Autodesk Inventor part; units mm, degrees
ref_plane "YZ Plane" through (0, 0, 0) normal (1, 0, 0) x (0, 1, 0)
ref_plane "XZ Plane" through (0, 0, 0) normal (0, 1, 0) x (-1, 0, 0)
ref_plane "XY Plane" through (0, 0, 0) normal (0, 0, 1) x (1, 0, 0)
sketch "Sketch1" plane through (0, 0, 0) normal (0, 0, 1) x (1, 0, 0)
  circle A0 centre (0, 0) radius 22
  dimension "d0" = 44
extrude "Extrusion1" add sketch "Sketch1" along normal blind 2
sketch "Sketch2" plane through (0, 0, 2) normal (0, 0, 1) x (1, 0, 0)
  line L0 (-15, 0) -> (15, 0) construction
  point P0 (0, 0)
  point P1 (0, 0)
  dimension "d3" = 30
hole "Hole1" at (-15, 0, 2) at (15, 0, 2) direction (0, 0, -1) diameter 3.4 end through all
sketch "Sketch3" plane through (0, 0, 2) normal (0, 0, 1) x (1, 0, 0)
  line L0 (-9, 15) -> (9, 15)
  line L1 (9, 15) -> (9, -15)
  line L2 (9, -15) -> (-9, -15)
  line L3 (-9, -15) -> (-9, 15)
  line L4 (7.2, 13.2) -> (-7.2, 13.2)
  line L5 (-7.2, 13.2) -> (-7.2, -13.2)
  line L6 (-7.2, -13.2) -> (7.2, -13.2)
  line L7 (7.2, -13.2) -> (7.2, 13.2)
  point P0 (0, 0)
  point P1 (9, 0)
  point P2 (0, 15)
  dimension "d11" = 30
  dimension "d12" = 18
  dimension "d13" = 1.8
extrude "Extrusion2" cut sketch "Sketch3" against normal blind 2 contours L7 L6 L5 L4
extrude "Extrusion3" add sketch "Sketch3" along normal blind 20
sketch "Sketch4" plane through (0, 0, 22) normal (0, 0, 1) x (1, 0, 0)
  line L0 (-9, -15) -> (9, -15)
  line L1 (9, -15) -> (9, 15)
  line L2 (9, 15) -> (-9, 15)
  line L3 (-9, 15) -> (-9, -15)
  line L4 (7.2, 13.2) -> (7.2, -13.2)
  line L5 (7.2, -13.2) -> (-7.2, -13.2)
  line L6 (-7.2, -13.2) -> (-7.2, 13.2)
  line L7 (-7.2, 13.2) -> (7.2, 13.2)
  point P0 (0, 0)
extrude "Extrusion4" add sketch "Sketch4" against normal blind 5 contours L4 L5 L6 L7
sketch "Sketch5" plane through (0, 0, 22) normal (0, 0, 1) x (1, 0, 0)
  point P0 (0, 0)
  point P1 (0, 0)
hole "Hole2" at (0, 0, 22) direction (0, 0, -1) diameter 5.1 end through all
fillet "Fillet1" radius 5 8 edges at (-7.2, -13.2, 8.5) (7.2, -13.2, 8.5) (-7.2, 13.2, 8.5) (7.2, 13.2, 8.5) (9, 15, 12) (-9, 15, 12) (-9, -15, 12) (9, -15, 12)
chamfer "Chamfer1" distance 5 angle 45 8 edges at (0, 13.2, 17) (-5.7355, 11.7355, 17) (-7.2, 0, 17) (-5.7355, -11.7355, 17) (0, -13.2, 17) (5.7355, -11.7355, 17) (7.2, 0, 17) (5.7355, 11.7355, 17)
chamfer "Chamfer2" distance 1 angle 45 24 edges at (0, 15, 22) (-7.5355, 13.5355, 22) (-9, 0, 22) (-7.5355, -13.5355, 22) (0, -15, 22) (7.5355, -13.5355, 22) (9, 0, 22) (7.5355, 13.5355, 22) (9, 0, 2) (7.5355, -13.5355, 2) (0, -15, 2) (-7.5355, -13.5355, 2) (-9, 0, 2) (-7.5355, 13.5355, 2) (0, 15, 2) (7.5355, 13.5355, 2) (7.2, 0, 0) (5.7355, 11.7355, 0) (0, 13.2, 0) (-5.7355, 11.7355, 0) (-7.2, 0, 0) (-5.7355, -11.7355, 0) (0, -13.2, 0) (5.7355, -11.7355, 0)
chamfer "Chamfer3" distance 0.4 angle 45 7 edges at (-22, 0, 2) (-22, 0, 0) (15, 1.7, 2) (-15, 1.7, 2) (-15, 1.7, 0) (15, 1.7, 0) (0, 2.55, 22)
properties part number "takumar-slit-led" material "ABS Plastic"
Verification items for the finished model (mm, model axes). A direction names the side the tool comes from. Round coordinates to 2 decimals unless told otherwise and drop trailing zeros. Loops run counter-clockwise (first coordinate to the right, second up) from the corner with the lowest first, then second, coordinate; pieces in that order, holes last. Notation, with made-up numbers: M 23,40.25 L 35,40.25 A21 ccw 35,44.25 Z; hole C -28,80 d4. An arc over 180 degrees is marked long. Write each question's results on one line, items separated by ' | '.
1) Section check B-B on z = 18.75. Record the boundary of the cut face in (x, y), then the cut area to 3 significant figures.
Checks:
outline: M -9,-10 A5 ccw -4,-15 L 4,-15 A5 ccw 9,-10 L 9,10 A5 ccw 4,15 L -4,15 A5 ccw -9,10 Z; hole C 0,0 d5.1 | area: 498 mm2
2) Scan lines: L1, parallel to Y at x = 2, z = 4.5; L2, parallel to Z at x = -12, y = 4; L3, parallel to Y at x = 15, z = 1. Record each from-to range of solid material in increasing order. Write a range as from..to.
Checks:
L1: y = -15..-13.2, 13.2..15 | L2: z = 0..2 | L3: y = -16.09..-1.7, 1.7..16.09
3) Access from +Z, -Z, +X, -X, +Y, -Y to the whole of each face (thin tool, end or side, straight path). Record for faces 5 (the flat face through (-9, 0, 12)), 6 (the flat face through (-4.7, -0.1, 14.5)), 7 (the cylindrical face through (-8, -13, 12)).
Checks:
face 5: +Z, -X, +Y, -Y | face 6: -Z | face 7: +Z, -X, -Y
4) Mould release check, pull along X, two halves, no side actions. Record for faces 1 (the cylindrical face through (7, -14, 12)), 2 (the conical face through (-7.778, 13.696, 2.715)), 3 (the flat face through (0.1, 15.5, 2.5)), 4 (the conical face through (4.012, -9.973, 14.465)): released by +X, released by -X, zero draft, split by the parting line, or undercut.
Checks:
face 1: released by +X | face 2: released by -X | face 3: zero draft | face 4: undercut
5) Section check C-C on y = 0. State how many separate pieces and enclosed holes the cut face has, then the cut area to 3 significant figures.
Checks:
separate pieces: 4 | enclosed holes: 0 | area: 187 mm2
6) Section check D-D on z = 8. Record the boundary of the cut face in (x, y).
Checks:
outline: M -9,-10 A5 ccw -4,-15 L 4,-15 A5 ccw 9,-10 L 9,10 A5 ccw 4,15 L -4,15 A5 ccw -9,10 Z; hole M -7.2,-8.2 A5 ccw -2.2,-13.2 L 2.2,-13.2 A5 ccw 7.2,-8.2 L 7.2,8.2 A5 ccw 2.2,13.2 L -2.2,13.2 A5 ccw -7.2,8.2 Z
7) Gauge pin test, flat ends, axial feed: P1, Ø12, axis at x = -9, z = 15.5, coming from the -Y side; P2, Ø5, axis at x = -0.5, y = -5.5, coming from the -Z side; P3, Ø9, axis at y = -2, z = 15.5, coming from the -X side. Record the tip position at first contact, or that the pin passes through.
Checks:
P1: stops at y = -15 | P2: stops at z = 16.2 | P3: stops at x = -9
